```python
from build123d import *

# Parameters (mm, degrees)
SKETCH2_R           = 4
BOSS_EXTRUDE1_DEPTH = 4


with BuildPart() as part:
    # Sketch2 → Boss-Extrude1 (new body)
    with BuildSketch(Plane(origin=(0, 0, 0), x_dir=(1, 0, 0), z_dir=(0, 1, 0))):
        Polygon((-65.617598228, 28.706575469), (-65.617598228, -111.293424531), (-45.617598228, -111.293424531), (-45.617598228, -115.293424531), (-5.617598228, -115.293424531), (-5.617598228, -111.293424531), (54.382401772, -111.293424531), (54.382401772, -115.293424531), (94.382401772, -115.293424531), (94.382401772, -111.293424531), (154.382401772, -111.293424531), (154.382401772, -115.293424531), (194.382401772, -115.293424531), (194.382401772, -111.293424531), (214.382401772, -111.293424531), (214.382401772, 28.706575469), (194.382401772, 28.706575469), (194.382401772, 32.706575469), (154.382401772, 32.706575469), (154.382401772, 28.706575469), (94.382401772, 28.706575469), (94.382401772, 32.706575469), (54.382401772, 32.706575469), (54.382401772, 28.706575469), (-5.617598228, 28.706575469), (-5.617598228, 32.706575469), (-45.617598228, 32.706575469), (-45.617598228, 28.706575469), align=None)
        with Locations(Location((-55.617598228, 12.706575469, 0), (0, 0, 270))):
            Circle(SKETCH2_R, mode=Mode.SUBTRACT)
        with Locations(Location((-55.617598228, -14.293424531, 0), (0, 0, 270))):
            Circle(SKETCH2_R, mode=Mode.SUBTRACT)
        with Locations(Location((-55.617598228, -41.293424531, 0), (0, 0, 270))):
            Circle(SKETCH2_R, mode=Mode.SUBTRACT)
        with Locations(Location((-55.617598228, -68.293424531, 0), (0, 0, 270))):
            Circle(SKETCH2_R, mode=Mode.SUBTRACT)
        with Locations(Location((-55.617598228, -95.293424531, 0), (0, 0, 270))):
            Circle(SKETCH2_R, mode=Mode.SUBTRACT)
        with Locations(Location((204.382401772, -95.293424531, 0), (0, 0, 270))):
            Circle(SKETCH2_R, mode=Mode.SUBTRACT)
        with Locations(Location((204.382401772, -68.293424531, 0), (0, 0, 270))):
            Circle(SKETCH2_R, mode=Mode.SUBTRACT)
        with Locations(Location((204.382401772, -41.293424531, 0), (0, 0, 270))):
            Circle(SKETCH2_R, mode=Mode.SUBTRACT)
        with Locations(Location((204.382401772, -14.293424531, 0), (0, 0, 270))):
            Circle(SKETCH2_R, mode=Mode.SUBTRACT)
        with Locations(Location((204.382401772, 12.706575469, 0), (0, 0, 270))):
            Circle(SKETCH2_R, mode=Mode.SUBTRACT)
        with Locations(Location((74.382401772, 12.706575469, 0), (0, 0, 270))):
            Circle(SKETCH2_R, mode=Mode.SUBTRACT)
        with BuildLine():
            Line((39.126697, 6.98825761), (-38.288984409, -28.616858167))
            ThreePointArc((-38.288984409, -28.616858167), (-39.985501487, -30.092867561), (-40.617598228, -32.250928644))
            Line((-40.617598228, -32.250928644), (-40.617598228, -86.964107845))
            ThreePointArc((-40.617598228, -86.964107845), (-38.005383219, -90.715647904), (-33.580571819, -89.567273339))
            Line((-33.580571819, -89.567273339), (43.835109591, 0.751021639))
            ThreePointArc((43.835109591, 0.751021639), (43.990577731, 5.764161935), (39.126697, 6.98825761))
        make_face(mode=Mode.SUBTRACT)
        with BuildLine():
            Line((-40.617598228, 19.706575469), (-40.617598228, -12.438434514))
            ThreePointArc((-40.617598228, -12.438434514), (-38.775659311, -15.806337773), (-34.946212047, -16.072504992))
            Line((-34.946212047, -16.072504992), (34.946212047, 16.072504992))
            ThreePointArc((34.946212047, 16.072504992), (37.182272725, 20.562063076), (33.274825866, 23.706575469))
            Line((33.274825866, 23.706575469), (-36.617598228, 23.706575469))
            ThreePointArc((-36.617598228, 23.706575469), (-39.446025353, 22.535002594), (-40.617598228, 19.706575469))
        make_face(mode=Mode.SUBTRACT)
        with BuildLine():
            Line((-26.049612497, -106.293424531), (16.328011378, -106.293424531))
            ThreePointArc((16.328011378, -106.293424531), (18.613731131, -105.576027951), (20.079567117, -103.681167137))
            Line((20.079567117, -103.681167137), (54.190855271, -11.46637295))
            ThreePointArc((54.190855271, -11.46637295), (52.897576456, -7.839367943), (49.099418661, -8.473191875))
            Line((49.099418661, -8.473191875), (-29.086638907, -99.690259037))
            ThreePointArc((-29.086638907, -99.690259037), (-29.683664091, -103.964851769), (-26.049612497, -106.293424531))
        make_face(mode=Mode.SUBTRACT)
        with BuildLine():
            Line((79.382401772, -15.979265858), (79.382401772, -102.293424531))
            ThreePointArc((79.382401772, -102.293424531), (80.553974647, -105.121851656), (83.382401772, -106.293424531))
            Line((83.382401772, -106.293424531), (113.244754244, -106.293424531))
            ThreePointArc((113.244754244, -106.293424531), (116.527357664, -104.579144283), (116.996309982, -100.905681925))
            Line((116.996309982, -100.905681925), (85.196068576, -14.938458903))
            ThreePointArc((85.196068576, -14.938458903), (81.853724371, -13.026216551), (79.382401772, -15.979265858))
        make_face(mode=Mode.SUBTRACT)
        with BuildLine():
            Line((35.5200493, -106.293424531), (65.382401772, -106.293424531))
            ThreePointArc((65.382401772, -106.293424531), (68.210828897, -105.121851656), (69.382401772, -102.293424531))
            Line((69.382401772, -102.293424531), (69.382401772, -15.979265858))
            ThreePointArc((69.382401772, -15.979265858), (66.911079173, -13.026216551), (63.568734968, -14.938458903))
            Line((63.568734968, -14.938458903), (31.768493562, -100.905681925))
            ThreePointArc((31.768493562, -100.905681925), (32.23744588, -104.579144283), (35.5200493, -106.293424531))
        make_face(mode=Mode.SUBTRACT)
        with BuildLine():
            Line((187.053787953, -28.616858167), (109.638106544, 6.98825761))
            ThreePointArc((109.638106544, 6.98825761), (104.774225813, 5.764161935), (104.929693953, 0.751021639))
            Line((104.929693953, 0.751021639), (182.345375363, -89.567273339))
            ThreePointArc((182.345375363, -89.567273339), (186.770186763, -90.715647904), (189.382401772, -86.964107845))
            Line((189.382401772, -86.964107845), (189.382401772, -32.250928644))
            ThreePointArc((189.382401772, -32.250928644), (188.750305031, -30.092867561), (187.053787953, -28.616858167))
        make_face(mode=Mode.SUBTRACT)
        with BuildLine():
            Line((185.382401772, 23.706575469), (115.489977678, 23.706575469))
            ThreePointArc((115.489977678, 23.706575469), (111.582530819, 20.562063076), (113.818591497, 16.072504992))
            Line((113.818591497, 16.072504992), (183.711015591, -16.072504992))
            ThreePointArc((183.711015591, -16.072504992), (187.540462855, -15.806337773), (189.382401772, -12.438434514))
            Line((189.382401772, -12.438434514), (189.382401772, 19.706575469))
            ThreePointArc((189.382401772, 19.706575469), (188.210828897, 22.535002594), (185.382401772, 23.706575469))
        make_face(mode=Mode.SUBTRACT)
        with BuildLine():
            Line((94.573948273, -11.46637295), (128.685236427, -103.681167137))
            ThreePointArc((128.685236427, -103.681167137), (130.151072413, -105.576027951), (132.436792166, -106.293424531))
            Line((132.436792166, -106.293424531), (174.814416041, -106.293424531))
            ThreePointArc((174.814416041, -106.293424531), (178.448467635, -103.964851769), (177.851442451, -99.690259037))
            Line((177.851442451, -99.690259037), (99.665384883, -8.473191875))
            ThreePointArc((99.665384883, -8.473191875), (95.867227088, -7.839367943), (94.573948273, -11.46637295))
        make_face(mode=Mode.SUBTRACT)
    extrude(amount=BOSS_EXTRUDE1_DEPTH)


solid = part.part
```
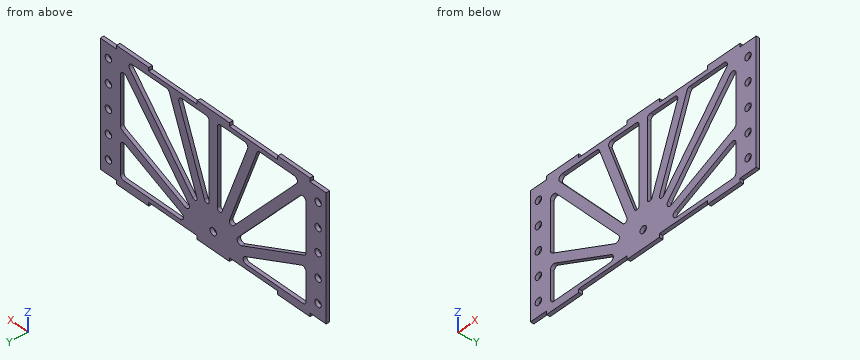
Input: part model. Units: mm. Frame: model coordinates. Give positions to 0.01 mm unless a question says otherwise; leave off trailing zeros. Order: outer loops, then holes, each group sorted by start corner. A loop starts at its lowest first (then second) coordinate and runs counter-clockwise, first axis right, second up. Notation, with made-up numbers: (40.25, 34.25) - (46.25, 34.25) arc R16 ccw to (46.25, 65.25) - close; hole circle Ø11 at (-25, 32). An arc over 180 degrees is marked (long way). Put each result on its own line as item: value.
Item 1: Contact query for flat-ended pins moving along their axis: pin 1 (2 mm diameter, centred on y = 2, z = -30.5, fed in from +X); pin 2 (1.5 mm diameter, centred on x = 109.5, y = 1.5, fed in from -Z). Output: stop coordinate, or through.
Found:
pin 1: stops at x = 194.38
pin 2: stops at z = -28.71
Item 2: Section query B-B, the plane z = 60. Return loops of the section in (x, y), then the cut area to 3 significant figures.
Found:
outline: (-65.62, 0) - (-40.62, 0) - (-40.62, 4) - (-65.62, 4) - close; (-8.24, 0) - (4.93, 0) - (4.93, 4) - (-8.24, 4) - close; (36.24, 0) - (46.9, 0) - (46.9, 4) - (36.24, 4) - close; (69.38, 0) - (79.38, 0) - (79.38, 4) - (69.38, 4) - close; (101.86, 0) - (112.53, 0) - (112.53, 4) - (101.86, 4) - close; (143.83, 0) - (157, 0) - (157, 4) - (143.83, 4) - close; (189.38, 0) - (214.38, 0) - (214.38, 4) - (189.38, 4) - close
area: 431 mm^2
Item 3: Section query A-A, the plane z = 3. Return loops of the section in (x, y), then the cut area to 3 significant figures.
Found:
outline: (-65.62, 0) - (-40.62, 0) - (-40.62, 4) - (-65.62, 4) - close; (-6.52, 0) - (17.41, 0) - (17.41, 4) - (-6.52, 4) - close; (40.62, 0) - (108.14, 0) - (108.14, 4) - (40.62, 4) - close; (131.36, 0) - (155.29, 0) - (155.29, 4) - (131.36, 4) - close; (189.38, 0) - (214.38, 0) - (214.38, 4) - (189.38, 4) - close
area: 662 mm^2
Item 4: Section query C-C, the plane y = 1.3. Count the separate pieces of the cut face and the enclosed holes in it, then the cut area to 3 significant figures.
Found:
separate pieces: 1
enclosed holes: 19
area: 19,400 mm^2
Item 5: Ray query, L1, parallel to Z at x = -30.5, y = 3.6; L2, parallel to X at y = 0.3, z = -21; L3, parallel to X at y = 0.4, z = -22. Return the intervals inside material, ascending. Write a range as from..to.
Found:
L1: z = -32.71..-23.71, 14.03..25.03, 85.97..115.29
L2: x = -65.62..-40.4, 37.06..111.7, 189.17..214.38
L3: x = -65.62..-39.89, 36.55..112.21, 188.66..214.38
